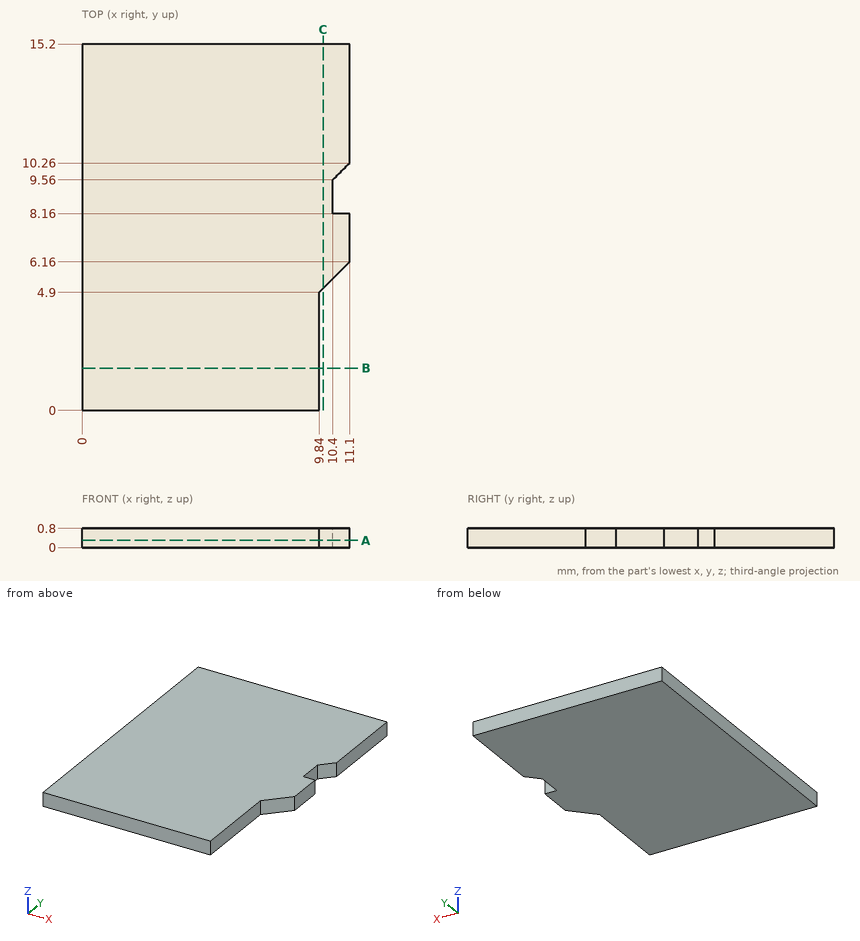
Study the drawing (mm; zero at the part's minimum x, y, z) and answer. Coordinates: 2 decimals unless noted, no trailing zeros. Write each loop counter-clockwise with the first axis right and the second up, starting at its lowest first coordinate (ties: lowest second). Pieces come first, ordered by that corner, then holes. Notation, with made-up numbers: (4.5, 1.5) - (60.5, 1.5) arc R36 ccw to (60.5, 35.5) - close; hole circle Ø2 at (38.25, 85.5). An arc over 180 degrees is marked (long way). Return JSON: item names as keys, results as strings. Group by question number.
1. A cutting plane is placed at B-B, the plane y = 1.75. Determine the outline of the cut face in (x, z), plus the area to 3 significant figures.
2. A cutting plane is placed at A-A, the plane z = 0.3. Determine the outline of the cut face in (x, y).
3. Straight lines are drawn through the part: L1, parallel to X at y = 9.5, z = 0.6; L2, parallel to X at y = 3, z = 0.15. For each, find the intervals that lie inside material, in ascending order.
4. A cutting plane is placed at C-C, the plane x = 10. Determine the outline of the cut face in (y, z), plus the area to 3 significant figures.
Ans:
{
 "1": {"outline": "(0, 0) - (9.84, 0) - (9.84, 0.8) - (0, 0.8) - close", "area": "7.87 mm²"},
 "2": {"outline": "(0, 0) - (9.84, 0) - (9.84, 4.9) - (11.1, 6.16) - (11.1, 8.16) - (10.4, 8.16) - (10.4, 9.56) - (11.1, 10.26) - (11.1, 15.2) - (0, 15.2) - close"},
 "3": {"L1": "0 to 10.4", "L2": "0 to 9.84"},
 "4": {"outline": "(5.06, 0) - (15.2, 0) - (15.2, 0.8) - (5.06, 0.8) - close", "area": "8.11 mm²"}
}
